Geometry check sheet. Reference: drawing and pictorial views, mm from the part's lowest x, y, z. A direction names the side the tool comes from. Round coordinates to 2 decimals unless told otherwise and drop trailing zeros. Order: outer loops, then holes, each group sorted by start corner. A loop starts at its lowest first (then second) coordinate and runs counter-clockwise, first axis right, second up.
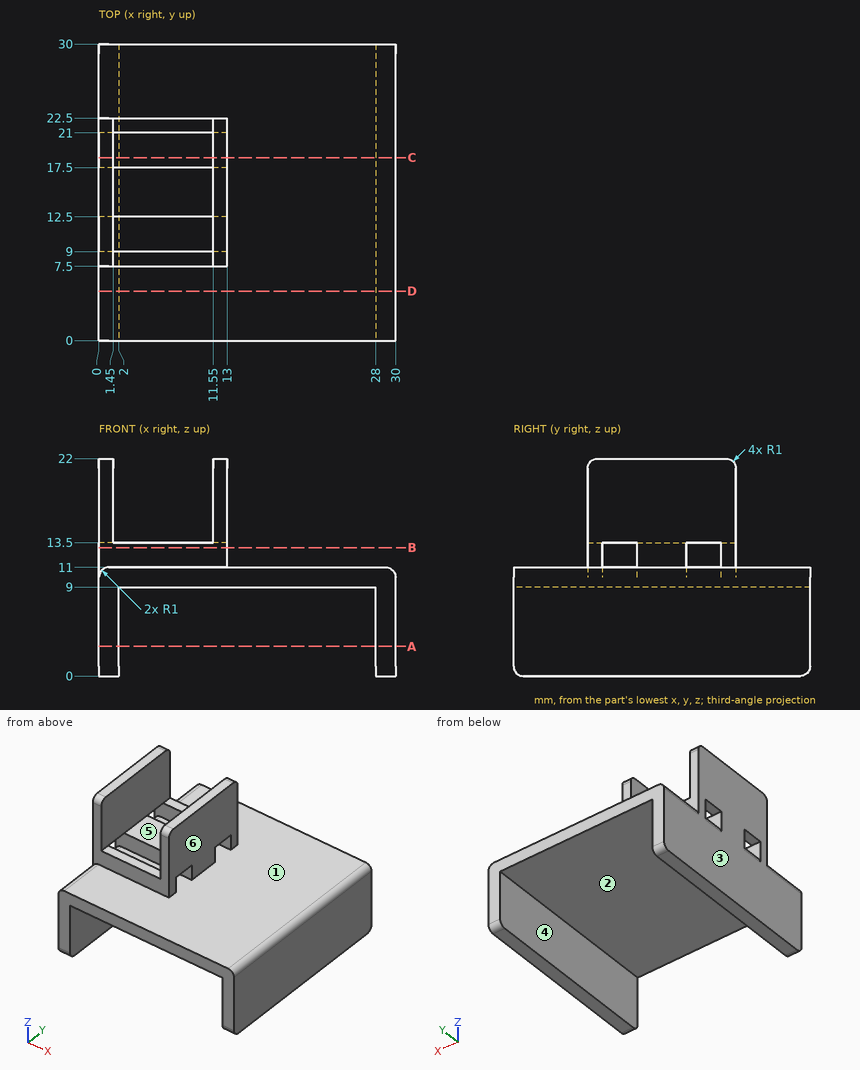
1) Tool access check on the marked faces 4, 5 and 6. Record the directions out of +Z, -Z, +X, -X, +Y, -Y that give a thin tool (end or side, any length) a straight path to the whole face; none if there is none.
2) Sectioned sample at D-D on y = 5. Record the cut outline in (x, z).
3) Sectioned sample at B-B on z = 13. Record the cut outline in (x, y).
4) Sectioned sample at C-C on y = 18.5. Record the cut outline in (x, z).
5) Draft check along X on the marked faces 1, 2 and 3. Enter one of: released by +X, released by -X, zero draft, split by the parting line, or undercut.
6) Scan lines: probe 1 along Y at (x, z) = (9.5, 12); probe 2 along X at (y, z) = (5.75, 6); probe 3 along X at (y, z) = (21.75, 15.25). Record each from-to range of solid material in increasing order.
7) Sectioned sample at A-A on z = 3. Record the cut outline in (x, y), then the cut area to 3 significant figures.
8) Go/stop test with flat-tipped pins: pin 1 Ø8 at (x, y) = (24, 16.5) entering from +Z; pin 2 Ø5.5 at (x, y) = (8, 15) entering from +Z; pin 3 Ø1.2 at (x, y) = (12, 11) entering from -Z; pin 4 Ø1 at (y, z) = (24, 19.5) entering from -X. Record where each tip stops, or that it passes through.
Returned:
1. face 4: -Z, +Y, -Y
1. face 5: +Z, +Y, -Y
1. face 6: +Z, +X, +Y, -Y
2. outline: (0, 0) - (2, 0) - (2, 9) - (28, 9) - (28, 0) - (30, 0) - (30, 10) arc R1 ccw to (29, 11) - (1, 11) arc R1 ccw to (0, 10) - close
3. outline: (0, 7.5) - (13, 7.5) - (13, 9) - (0, 9) - close; (0, 12.5) - (13, 12.5) - (13, 17.5) - (0, 17.5) - close; (0, 21) - (13, 21) - (13, 22.5) - (0, 22.5) - close
4. outline: (0, 0) - (2, 0) - (2, 9) - (28, 9) - (28, 0) - (30, 0) - (30, 10) arc R1 ccw to (29, 11) - (1, 11) arc R1 ccw to (0, 10) - close; (0, 13.5) - (1.45, 13.5) - (1.45, 22) - (0, 22) - close; (11.55, 13.5) - (13, 13.5) - (13, 22) - (11.55, 22) - close
5. face 1: zero draft
5. face 2: undercut
5. face 3: released by -X
6. probe 1: y = 7.5 to 9, 12.5 to 17.5, 21 to 22.5
6. probe 2: x = 0 to 2, 28 to 30
6. probe 3: x = 0 to 1.45, 11.55 to 13
7. outline: (0, 0) - (2, 0) - (2, 30) - (0, 30) - close; (28, 0) - (30, 0) - (30, 30) - (28, 30) - close
7. area: 120 mm2
8. pin 1: stops at z = 11
8. pin 2: stops at z = 13.5
8. pin 3: stops at z = 9
8. pin 4: passes through
